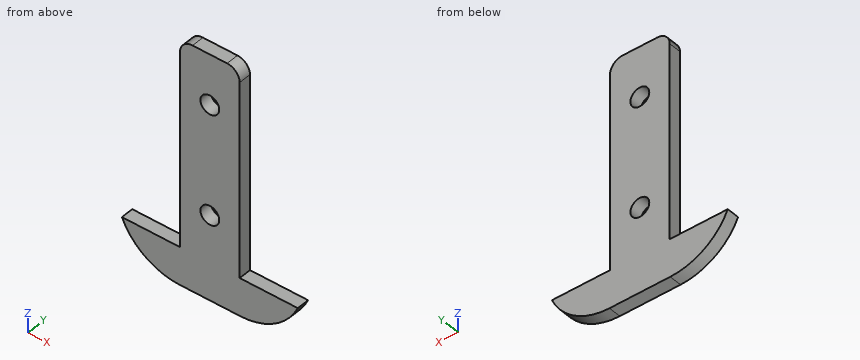
from build123d import *

# Parameters (mm, degrees)
SKETCH1_W           = 9.5
SKETCH1_H           = 33
SKETCH1_W_2         = 28
SKETCH1_H_2         = 6
BOSS_EXTRUDE2_DEPTH = 2
SKETCH2_R           = 1.5
CUT_EXTRUDE1_DEPTH  = 27.575364532
FILLET6_R           = 10
FILLET7_R           = 10
FILLET10_R          = 2


with BuildPart() as part:
    # Sketch1 → Boss-Extrude2 (new body)
    with BuildSketch(Plane(origin=(0, 0, 0), x_dir=(1, 0, 0), z_dir=(0, 1, 0))):
        Rectangle(SKETCH1_W, SKETCH1_H)
        with Locations((0, 19.5)):
            Rectangle(SKETCH1_W_2, SKETCH1_H_2)
    extrude(amount=BOSS_EXTRUDE2_DEPTH)

    # Sketch2 → Cut-Extrude1 (cut, through all)
    with BuildSketch(Plane.XZ):
        with Locations(Location((0, 8.5, 0), (0, 0, 270))):
            Circle(SKETCH2_R)
        with Locations(Location((0, -9, 0), (0, 0, 270))):
            Circle(SKETCH2_R)
    extrude(amount=-CUT_EXTRUDE1_DEPTH, mode=Mode.SUBTRACT)

    # Fillet6
    # the kernel refuses this fillet: 10 mm, written as the material it takes off along each edge
    with BuildSketch(Plane(origin=(14, -22.912878475, -22.5), x_dir=(-1, 0, 0), z_dir=(0, 1, 0))) as fillet6_piece_1:
        with BuildLine():
            CenterArc((9.16515139, 10), FILLET6_R, 203.578178478, 66.421821522)
            Line((0, 6), (-0.183303028, 5.92))
            ThreePointArc((-0.183303028, 5.92), (-0.2, 3), (-0.2, 0))
            Line((-0.2, 0), (0, -0.2))
            Line((0, -0.2), (9.16515139, -0.2))
            Line((9.16515139, -0.2), (9.16515139, 0))
        make_face()
    extrude(amount=47.82575695, mode=Mode.SUBTRACT)

    # Fillet7
    # the kernel refuses this fillet: 10 mm, written as the material it takes off along each edge
    with BuildSketch(Plane(origin=(-14, -22.912878475, -22.5), x_dir=(0, 0, 1), z_dir=(0, 1, 0))) as fillet7_piece_1:
        with BuildLine():
            CenterArc((10, 9.16515139), FILLET7_R, 180, 66.421821522)
            Line((0, 9.16515139), (-0.2, 9.16515139))
            Line((-0.2, 9.16515139), (-0.2, 0))
            Line((-0.2, 0), (0, -0.2))
            ThreePointArc((0, -0.2), (3, -0.2), (5.92, -0.183303028))
            Line((5.92, -0.183303028), (6, 0))
        make_face()
    extrude(amount=47.82575695, mode=Mode.SUBTRACT)

    # Fillet10
    fillet10_edges = [part.edges().sort_by_distance(p)[0] for p in [
        (4.75, 1, 16.5),
        (-4.75, 1, 16.5),
    ]]
    fillet(fillet10_edges, radius=FILLET10_R)


solid = part.part
Geometry check sheet. Reference: the model listing, model coordinates, mm. Round coordinates to 2 decimals unless told otherwise and drop trailing zeros. Loops run counter-clockwise (first coordinate to the right, second up) from the corner with the lowest first, then second, coordinate; pieces in that order, holes last. Notation, with made-up numbers: (-22, 88.5) -> (25, 88.5) arc R16 cw to (25, 117.5) -> close; hole circle Ø10 at (-9.5, -37). An arc over 180 degrees is marked (long way). Answer as a JSON object with one key per item and string values. Group by question number.
Item 1: Cross-section at D-D, the plane x = 9. Record the cut outline in (y, z).
Item 2: Cross-section at C-C, the plane y = 1.15. Record the cut outline in (x, z).
Item 3: Depth check by flat-ended pin: pin 1 Ø1 at (x, y) = (-10, 1.5) entering from -Z; pin 2 Ø12 at (x, z) = (-11, -12.5) entering from +Y; pin 3 Ø1 at (y, z) = (0.5, -4) entering from +X. Enter the tip coordinate at first touch or a pass-through.
Item 4: Thickness scan on line 1 along X through (y, z) = (1.3, 8.5); line 2 along Z through (x, y) = (-0.25, 0.2); line 3 along X through (y, z) = (1.7, -12.5). Record the ranges inside material, lowest first.
Item 5: Cross-section at B-B, the plane x = 0. Record the cut outline in (y, z).
Item 6: Cross-section at A-A, the plane z = 8.5. Record the cut outline in (x, y).
Determined:
{
 "1": {"outline": "(0, -21.59) -> (2, -21.59) -> (2, -16.5) -> (0, -16.5) -> close"},
 "2": {"outline": "(-14, -16.5) arc R10 ccw to (-4.83, -22.5) -> (4.83, -22.5) arc R10 ccw to (14, -16.5) -> (4.75, -16.5) -> (4.75, 14.5) arc R2 ccw to (2.75, 16.5) -> (-2.75, 16.5) arc R2 ccw to (-4.75, 14.5) -> (-4.75, -16.5) -> close; hole circle Ø3 at (0, -9); hole circle Ø3 at (0, 8.5)"},
 "3": {"pin 1": "stops at z = -21.35", "pin 2": "stops at y = 2", "pin 3": "stops at x = 4.75"},
 "4": {"line 1": "x = -4.75 to -1.5, 1.5 to 4.75", "line 2": "z = -22.5 to -10.48, -7.52 to 7.02, 9.98 to 16.5", "line 3": "x = -4.75 to 4.75"},
 "5": {"outline": "(0, -22.5) -> (2, -22.5) -> (2, -10.5) -> (0, -10.5) -> close; (0, -7.5) -> (2, -7.5) -> (2, 7) -> (0, 7) -> close; (0, 10) -> (2, 10) -> (2, 16.5) -> (0, 16.5) -> close"},
 "6": {"outline": "(-4.75, 0) -> (-1.5, 0) -> (-1.5, 2) -> (-4.75, 2) -> close; (1.5, 0) -> (4.75, 0) -> (4.75, 2) -> (1.5, 2) -> close"}
}
